The listing builds one solid part. Answer for the finished solid, in the listing's coordinates (mm). A direction names the side the tool comes from. Round coordinates to 2 decimals unless told otherwise and drop trailing zeros. Write each loop counter-clockwise with the first axis right and the second up, starting at its lowest first coordinate (ties: lowest second). Pieces come first, ordered by that corner, then holes.
from build123d import *

# Parameters (mm, degrees)
F0_W     = 79.766176641
F0_H     = 52.5435172021
F1_DEPTH = 12.7
F2_W     = 27.8192292899
F2_H     = 14.4076673314
F2_H_2   = 14.4076794386
F3_DEPTH = 12.7
F5_DEPTH = 12.7


with BuildPart() as f1:
    # F0 (on Top) → F1 (new body)
    with BuildSketch(Plane.XY):
        with Locations((39.8830883205, 26.2717586011)):
            Rectangle(F0_W, F0_H)
    extrude(amount=F1_DEPTH)

    # F2 (on face) → F3 (join)
    with BuildSketch(Plane.XY.offset(12.7)):
        Polygon((17.6650751382, 52.5435172021), (0, 52.5435172021), (0, 0), (17.6650751382, 0), (17.6650751382, 14.4076673314), (17.6650751382, 38.1358377635), align=None)
        with Locations((31.5746897832, 7.2038336657)):
            Rectangle(F2_W, F2_H)
        with Locations((31.5746897832, 45.3396774828)):
            Rectangle(F2_W, F2_H_2)
    extrude(amount=F3_DEPTH)

    # F4 (on face) → F5 (join)
    with BuildSketch(Plane.XY.offset(25.4)):
        Polygon((17.6650751382, 52.5435172021), (0, 52.5435172021), (0, 0), (17.6650751382, 0), (17.6650751382, 14.4076673314), (17.6650751382, 38.1358377635), align=None)
    extrude(amount=F5_DEPTH)


solid = f1.part
1. For a pull along Y with two mould halves and no side action, classify faces 1 (the face through (30, 0, 15)), 2 (the face through (31, 38.136, 19)), 3 (the face through (0, 27, 19)) as released by +Y, released by -Y, zero draft, split by the parting line, or undercut.
Geometry says:
face 1: released by -Y
face 2: undercut
face 3: zero draft
2. Given pin 1 (6.5 mm diameter, centred on y = 46, z = 18.5, fed in from +X); pin 2 (1.5 mm diameter, centred on x = 42.5, z = 27, fed in from +Y); pin 3 (11.5 mm diameter, centred on x = 34, y = 5, fed in from +Z), each flat-ended and moving along its own axis, determine where each tip first touches the part or whether it passes through.
Geometry says:
pin 1: stops at x = 45.48
pin 2: passes through
pin 3: stops at z = 25.4
3. Straight lines are drawn through the part: line 1 along X through (y, z) = (23, 20); line 2 along Y through (x, z) = (29.5, 22); line 3 along X through (y, z) = (44.5, 13). For each, find the intervals that lie inside material, in ascending order.
Geometry says:
line 1: x = 0 to 17.67
line 2: y = 0 to 14.41, 38.14 to 52.54
line 3: x = 0 to 45.48
4. Section D-D on z = 32 is taken. Determine the outline of the cut face in (x, y), plus the area to 3 significant figures.
Geometry says:
outline: (0, 0) - (17.67, 0) - (17.67, 52.54) - (0, 52.54) - close
area: 928 mm2
5. A tool of negligible diameter and unlimited length cuts with its end or side. For faces 4 (the face through (31, 14.408, 19)), 5 (the face through (9, 27, 38.1)), 6 (the face through (45.484, 7, 19)), from which of +Z, -Z, +X, -X, +Y, -Y can it reach the whole face along a straight path? Write none if from no direction.
Geometry says:
face 4: +Z, +X
face 5: +Z, +X, -X, +Y, -Y
face 6: +Z, +X, +Y, -Y
6. Section B-B on y = 24.5 is taken. Determine the outline of the cut face in (x, z).
Geometry says:
outline: (0, 0) - (79.77, 0) - (79.77, 12.7) - (17.67, 12.7) - (17.67, 38.1) - (0, 38.1) - close
7. Section A-A on x = 19.5 is taken. Determine the outline of the cut face in (y, z), plus the area to 3 significant figures.
Geometry says:
outline: (0, 0) - (52.54, 0) - (52.54, 25.4) - (38.14, 25.4) - (38.14, 12.7) - (14.41, 12.7) - (14.41, 25.4) - (0, 25.4) - close
area: 1,030 mm2
8. Section C-C on z = 17 is taken. Determine the outline of the cut face in (x, y), plus the area to 3 significant figures.
Geometry says:
outline: (0, 0) - (45.48, 0) - (45.48, 14.41) - (17.67, 14.41) - (17.67, 38.14) - (45.48, 38.14) - (45.48, 52.54) - (0, 52.54) - close
area: 1,730 mm2
